Input: part model. Units: mm. Frame: model coordinates. A direction names the side the tool comes from. Give positions to 0.01 mm unless a question says otherwise; leave off trailing zeros. Loops run counter-clockwise (first coordinate to the right, second up) from the corner with the lowest first, then second, coordinate; pieces in that order, holes last. Notation, with made-up numbers: M -0.75,80 L 10.25,80 A16 ccw 10.25,100 Z; hole C -39,88 d6. An arc over 180 degrees is marked long. Answer as a JSON object with one key per item and string values. Group by question number.
```python
from build123d import *

# Parameters (mm, degrees)
F0_R     = 16.5
F0_R_2   = 11.5
F1_DEPTH = 25
F2_W     = 33
F2_H     = 50
F3_DEPTH = 20
F5_D     = 8.4
F5_DEPTH = 25.001
F6_D     = 8.4
F7_R     = 5


with BuildPart() as f1:
    # F0 (on Top) → F1 (new body)
    with BuildSketch(Plane.XY):
        Circle(F0_R)
        Circle(F0_R_2, mode=Mode.SUBTRACT)
    extrude(amount=F1_DEPTH)

    # F2 (on Top) → F3 (join)
    with BuildSketch(Plane.XY):
        Rectangle(F2_W, F2_H)
    extrude(amount=-F3_DEPTH)

    # F5 (through all, one way)
    with BuildSketch(Plane(origin=(0, 0, 0), x_dir=(1, 0, 0), z_dir=(0, 1, 0))):
        with Locations((0, 10.8142616227)):
            Circle(F5_D / 2)
    extrude(amount=-F5_DEPTH, mode=Mode.SUBTRACT)

    # F6 (through all)
    with Locations(Plane.XZ):
        with Locations((0, -10.8142616227)):
            Hole(F6_D / 2)

    # F7
    f7_edges = [f1.edges().sort_by_distance(p)[0] for p in [
        (0, 25, -20),
        (-16.5, 0, -20),
        (0, -25, -20),
        (16.5, 0, -20),
        (-16.5, 25, -10),
        (16.5, 25, -10),
        (16.5, -25, -10),
        (-16.5, -25, -10),
    ]]
    fillet(f7_edges, radius=F7_R)


solid = f1.part
```
1. Mould query, pull axis Y, two halves, no side actions, for faces 4 (the cylindrical face through (6, -24, -18)), 5 (the flat face through (0, 0, 0)), 6 (the cylindrical face through (-1.5, 11.4, 12.3)), 7 (the cylindrical face through (15, 0.28, -18.57)). Classes: pulls with the +Y half, pulls with the -Y half, needs draft (parallel to the pull), parting line crosses it, or undercut.
2. Section C-C (y = 7.5). Output: boundary loops of the cut face in (x, z).
3. First-contact query: P1, Ø13.5, axis at x = 0, z = -10.81, coming from the -Y side; P2, Ø8, axis at x = -4.5, z = 14.5, coming from the +Y side; P3, Ø1, axis at y = 18.5, z = 5, coming from the -X side; P4, Ø4, axis at x = 11, z = 13.5, coming from the -Y side. Flat tips, straight axial feed; report the tip coordinate or a pass-through.
4. Section B-B (x = 9). Output: boundary loops of the cut face in (y, z).
5. Material intervals for L1, parallel to Y at x = 0, z = 7.5; L2, parallel to Z at x = 0, y = 16; L3, parallel to Z at x = 8, y = 19.5, sorted ascending.
6. Reachability of faces 1 (the flat face through (0, 18, 0)), 2 (the cylindrical face through (15.24, -6.32, 12.32)), 3 (the flat face through (0, -18, 0)) from +Z, -Z, +X, -X, +Y, -Y: full face, straight path, thin tool, end or side. Return the list, or none.
7. Section D-D (x = -6). Output: boundary loops of the cut face in (y, z), then the cut area to 3 significant figures.
Geometry results:
{
 "1": {"face 4": "pulls with the -Y half", "face 5": "undercut", "face 6": "undercut", "face 7": "needs draft"},
 "2": {"outline": "M -16.5,-15 A5 ccw -11.5,-20 L 11.5,-20 A5 ccw 16.5,-15 L 16.5,0 L 14.7,0 L 14.7,25 L 8.72,25 L 8.72,0 L -8.72,0 L -8.72,25 L -14.7,25 L -14.7,0 L -16.5,0 Z; hole C 0,-10.81 d8.4"},
 "3": {"P1": "y = -25", "P2": "y = 16.49", "P3": "through", "P4": "y = -13.83"},
 "4": {"outline": "M -25,-15 A5 ccw -20,-20 L 20,-20 A5 ccw 25,-15 L 25,0 L 13.83,0 L 13.83,25 L 7.16,25 L 7.16,0 L -7.16,0 L -7.16,25 L -13.83,25 L -13.83,0 L -25,0 Z"},
 "5": {"L1": "-16.5 to -11.5, 11.5 to 16.5", "L2": "-20 to -15.01, -6.61 to 25", "L3": "-20 to 0"},
 "6": {"face 1": "+Z, +Y", "face 2": "+Z", "face 3": "+Z, -Y"},
 "7": {"outline": "M -25,-15 A5 ccw -20,-20 L 20,-20 A5 ccw 25,-15 L 25,0 L 15.37,0 L 15.37,25 L 9.81,25 L 9.81,0 L -9.81,0 L -9.81,25 L -15.37,25 L -15.37,0 L -25,0 Z", "area": "1,270 mm2"}
}
